Job drawing, mm, ordinate dimensions from the low corner. One solid piece. A direction names the side the tool comes from. Give positions to 0.01 mm unless a question says otherwise; leave off trailing zeros. Loops run counter-clockwise (first coordinate to the right, second up) from the corner with the lowest first, then second, coordinate; pieces in that order, holes last.
Item 1: Probe probe 1 along X at (y, z) = (29, 4.25); probe 2 along X at (y, z) = (46.5, 12); probe 3 along Y at (x, z) = (16, 12.75). List the from-to ranges inside material, lowest first.
Item 2: Saw through at D-D on y = 20.5. Give the cut face in (x, z), plus the area to 3 significant figures.
Item 3: Saw through at A-A on z = 3.75. Give the cut face in (x, y) (3 decimals).
Item 4: Saw through at B-B on y = 33.5. Give the cut face in (x, z), plus the area to 3 significant figures.
Item 5: Which spindle directions (+Z, -Z, +X, -X, +Y, -Y) get a long thin tool onto all of the face, cutting with end or side? Do the marked faces 1, 2 and 3. Say none if no direction does.
Item 6: Saw through at C-C on x = 9.5. Give the cut face in (y, z).
Item 7: Drop flat-ended pins along their axis: P1, Ø6, axis at x = 36.5, z = 7, coming from the +Y side; P2, Ø1, axis at x = 43, z = 6.5, coming from the -Y side; P3, Ø5, axis at x = 73, z = 1.5, coming from the +Y side. Give the stop position or say it passes through.
Item 8: Mould opens along X. For the marked faces 4, 5, 6 and 7 say: released by +X, released by -X, zero draft, split by the parting line, or undercut.
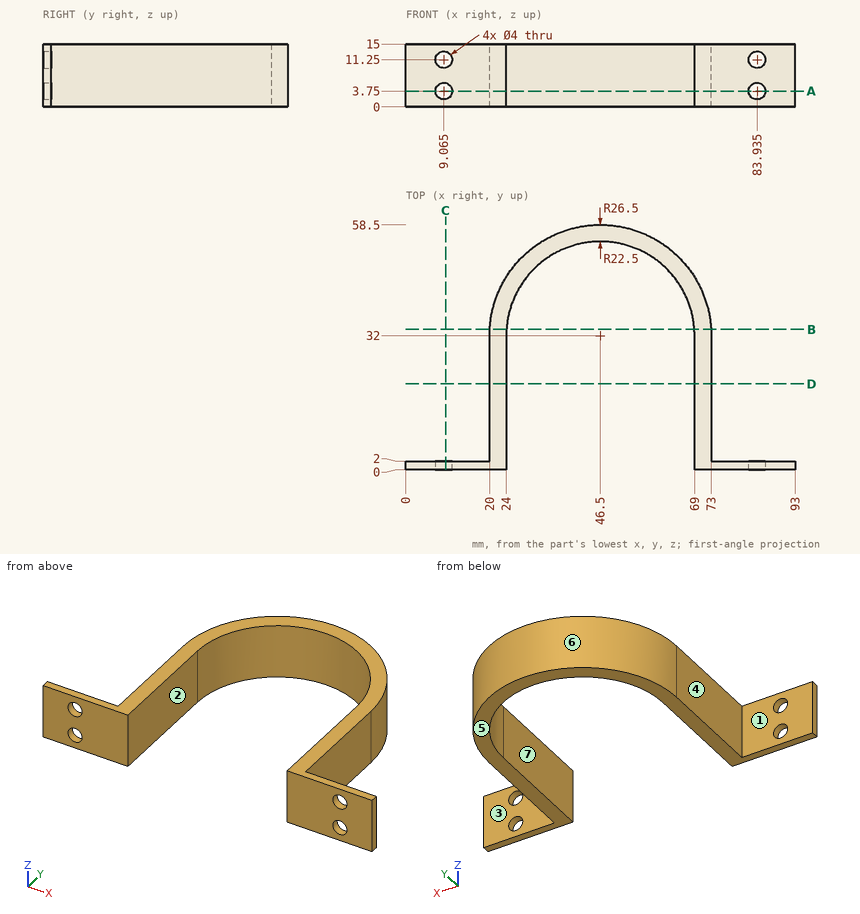
Results below:
1. probe 1: x = 20 to 24, 69 to 73
1. probe 2: x = 24.32 to 29.3, 63.7 to 68.68
1. probe 3: y = 0 to 2
2. outline: (20, 0) - (24, 0) - (24, 15) - (20, 15) - close; (69, 0) - (73, 0) - (73, 15) - (69, 15) - close
2. area: 120 mm2
3. outline: (0, 0) - (7.065, 0) - (7.065, 2) - (0, 2) - close; (11.065, 0) - (24, 0) - (24, 32) arc R22.5 cw to (69, 32) - (69, 0) - (81.935, 0) - (81.935, 2) - (73, 2) - (73, 32) arc R26.5 ccw to (20, 32) - (20, 2) - (11.065, 2) - close; (85.935, 0) - (93, 0) - (93, 2) - (85.935, 2) - close
4. outline: (20.04, 0) - (24.05, 0) - (24.05, 15) - (20.04, 15) - close; (68.95, 0) - (72.96, 0) - (72.96, 15) - (68.95, 15) - close
4. area: 120 mm2
5. face 1: +Z, -Z, -X, +Y
5. face 2: +Z, -Z, -Y
5. face 3: +Z, -Z, +X, +Y
6. outline: (0, 0) - (2, 0) - (2, 1.8) - (0, 1.8) - close; (0, 5.7) - (2, 5.7) - (2, 9.3) - (0, 9.3) - close; (0, 13.2) - (2, 13.2) - (2, 15) - (0, 15) - close
7. P1: stops at y = 57.56
7. P2: stops at y = 54.14
7. P3: stops at y = 43.24
8. face 4: released by -X
8. face 5: zero draft
8. face 6: split by the parting line
8. face 7: undercut
